Geometry: final body of the model. Coordinates: model frame, mm. A direction names the side the tool comes from. Coordinates: 2 decimals unless noted, no trailing zeros. Order: outer loops, then holes, each group sorted by start corner. A loop starts at its lowest first (then second) coordinate and runs counter-clockwise, first axis right, second up. Notation, with made-up numbers: (-9, -5.5) - (37, -5.5) arc R25 cw to (37, 29.5) - close; hole circle Ø6 at (-16.75, -9). An arc over 180 degrees is marked (long way). Use a Markdown table: item, result. Add a question column.
```python
from build123d import *

# Parameters (mm, degrees)
SKETCH1_R           = 95
BOSS_EXTRUDE1_DEPTH = 20
SKETCH2_R           = 6
CUT_EXTRUDE1_DEPTH  = 20
SKETCH5_R           = 45
BOSS_EXTRUDE3_DEPTH = 55
CUT_EXTRUDE2_DEPTH  = 75


with BuildPart() as part:
    # Sketch1 → Boss-Extrude1 (new body)
    with BuildSketch(Plane.XY):
        Circle(SKETCH1_R)
    extrude(amount=BOSS_EXTRUDE1_DEPTH)

    # Sketch2 → Cut-Extrude1 (cut)
    with BuildSketch(Plane.XY.offset(20)):
        with Locations((0, 70)):
            Circle(SKETCH2_R)
        with Locations((70, 0)):
            Circle(SKETCH2_R)
        with Locations(Location((0, -70, 0), (0, 0, 180))):
            Circle(SKETCH2_R)
        with Locations(Location((-70, 0, 0), (0, 0, 180))):
            Circle(SKETCH2_R)
    extrude(amount=-CUT_EXTRUDE1_DEPTH, mode=Mode.SUBTRACT)

    # Sketch5 → Boss-Extrude3 (add)
    with BuildSketch(Plane(origin=(0, 0, 0), x_dir=(-1, 0, 0), z_dir=(0, 0, -1))):
        with Locations(Location((0, 0, 0), (0, 0, 180))):
            Circle(SKETCH5_R)
    extrude(amount=BOSS_EXTRUDE3_DEPTH)

    # Sketch3 → Cut-Extrude2 (cut)
    with BuildSketch(Plane.XY.offset(20)):
        with BuildLine():
            Line((-6.940265993, 22.474071895), (-6.940265993, 21.402866816))
            ThreePointArc((-6.940265993, 21.402866816), (-0.062853214, -22.49991221), (7.059734007, 21.363757997))
            Line((7.059734007, 21.363757997), (7.059734007, 22.474071895))
            Line((7.059734007, 22.474071895), (7.059734007, 25.374071895))
            Line((7.059734007, 25.374071895), (-6.940265993, 25.374071895))
            Line((-6.940265993, 25.374071895), (-6.940265993, 22.474071895))
        make_face()
    extrude(amount=-CUT_EXTRUDE2_DEPTH, mode=Mode.SUBTRACT)


solid = part.part
```
1) First-contact query: pin 1 (6 mm diameter, centred on y = -64, z = 8, fed in from -X); pin 2 (14 mm diameter, centred on x = 0, y = -70, fed in from -Z); pin 3 (2 mm diameter, centred on y = 24, z = -3.5, fed in from +X). Flat tips, straight axial feed; report the tip coordinate or a pass-through.
2) Section query D-D (x = -70). Return the cut outline in (y, z), and give its area (3 significant figures).
3) Section query A-A (x = 0). Return the cut outline in (y, z).
4) Section query C-C (z = -15). Return the cut outline in (x, y).
5) Draft query along X for faces 1 (the flat face through (20, -20, 20)), 2 (the cylindrical face through (-20.59, -92.74, 9.86)), 3 (the cylindrical face through (0.78, -75.95, 10.14)). Return one class per face: released by +X, released by -X, zero draft, split by the parting line, or undercut.
6) Line query: line 1 (Y direction, x = 0, z = 7.25); line 2 (Y direction, x = 0, z = -31.5); line 3 (Z direction, x = 2.5, y = 61). Output: solid intervals per line, ascending. Write a range as from..to.
7) Section query B-B (y = 0). Return the cut outline in (x, z), and give its area (4 significant figures).
8) Access query for faces 4 (the flat face through (9, -21, -55)), 5 (the flat face through (0, 25.374, -17)), 6 (the flat face through (41, -20, 0)). Directions: +Z, -Z, +X, -X, +Y, -Y. A direction counts if a zero-diameter tool reaches every point of the face in a straight line with its end or side. Return the directions, or none.
From the geometry:
| question | item | result |
|---|---|---|
| 1 | pin 1 | stops at x = -72.83 |
| 1 | pin 2 | stops at z = 0 |
| 1 | pin 3 | stops at x = 38.68 |
| 2 | outline | (-64.23, 0) - (-6, 0) - (-6, 20) - (-64.23, 20) - close; (6, 0) - (64.23, 0) - (64.23, 20) - (6, 20) - close |
| 2 | area | 2,330 mm^2 |
| 3 | outline | (-95, 0) - (-76, 0) - (-76, 20) - (-95, 20) - close; (-64, 0) - (-45, 0) - (-45, -55) - (-22.5, -55) - (-22.5, 20) - (-64, 20) - close; (25.37, -55) - (45, -55) - (45, 0) - (64, 0) - (64, 20) - (25.37, 20) - close; (76, 0) - (95, 0) - (95, 20) - (76, 20) - close |
| 4 | outline | circle Ø90 at (0, 0); hole (-6.94, 21.4) arc R22.5 ccw (long way) to (7.06, 21.36) - (7.06, 25.37) - (-6.94, 25.37) - close |
| 5 | face 1 | zero draft |
| 5 | face 2 | split by the parting line |
| 5 | face 3 | undercut |
| 6 | line 1 | y = -95..-76, -64..-22.5, 25.37..64, 76..95 |
| 6 | line 2 | y = -45..-22.5, 25.37..45 |
| 6 | line 3 | z = 0..20 |
| 7 | outline | (-95, 0) - (-76, 0) - (-76, 20) - (-95, 20) - close; (-64, 0) - (-45, 0) - (-45, -55) - (-22.5, -55) - (-22.5, 20) - (-64, 20) - close; (22.5, -55) - (45, -55) - (45, 0) - (64, 0) - (64, 20) - (22.5, 20) - close; (76, 0) - (95, 0) - (95, 20) - (76, 20) - close |
| 7 | area | 4,895 mm^2 |
| 8 | face 4 | -Z, +X, -X, +Y, -Y |
| 8 | face 5 | +Z, -Z |
| 8 | face 6 | -Z |
